For this review, take the finished solid that the model builds, in its own axes (mm). A direction names the side the tool comes from. Coordinates: 2 decimals unless noted, no trailing zeros. Loops run counter-clockwise (first coordinate to the right, second up) from the corner with the lowest first, then second, coordinate; pieces in that order, holes last.
1. Mouldability with a two-part tool opening along Y and no side actions: class faces 3 (the face through (57, 61, 3.2)), 4 (the face through (130.22, 2.99, 1.58)), 5 (the face through (-31.069, 93.114, 1.578)), 6 (the face through (96.05, 4.46, 1.58)) as pulls with the +Y half, pulls with the -Y half, needs draft (parallel to the pull), parting line crosses it, or undercut.
2. Take a section at B-B, the plane y = 3.81. State the section outline as (x, z) points, then the cut area to 3 significant figures.
3. Take a section at C-C, the plane x = 108.5. State the section outline as (y, z) points, then the cut area to 3 significant figures.
4. To check wall thickness, follow probe 1 along Y at (x, z) = (100.5, 2.95); probe 2 along X at (y, z) = (28.5, 1.3); probe 3 along Y at (x, z) = (63, 0.5). State the ranges of each line that lie inside material, in increasing order.
5. Clearance check with a flat-ended pin moving along its axis: P1, Ø1, axis at x = 13.5, z = 1, coming from the +Y side. State where the tip first meets the part, or that it passes through.
6. Machinability: for faces 1 (the face through (-11.48, 3.11, 1.58)), 2 (the face through (72.58, 67.22, 1.62)), which of the approach directions +Z, -Z, +X, -X, +Y, -Y give a long, thin tool a straight path to every point of the face, cutting with its end or side? Answer none if there is none.
7. Take a section at D-D, the plane x = 12.5. State the section outline as (y, z) points, then the cut area to 3 significant figures.
8. Take a section at A-A, the plane x = 81. State the section outline as (y, z) points, then the cut area to 3 significant figures.
```python
from build123d import *

# Parameters (mm, degrees)
SKETCH1_R           = 3.429
SKETCH1_R_2         = 2.54
BOSS_EXTRUDE1_DEPTH = 3.2004
SKETCH2_R           = 2.159
CUT_EXTRUDE1_DEPTH  = 3.2004
CUT_EXTRUDE8_DEPTH  = 3.2004
SKETCH11_W          = 107.95
SKETCH11_H          = 3.2512
CUT_EXTRUDE9_DEPTH  = 3.2004
SKETCH12_R          = 1.1303
CUT_EXTRUDE11_DEPTH = 3.2004
SKETCH13_R          = 2.2479
CUT_EXTRUDE12_DEPTH = 3.2004
BOSS_EXTRUDE2_DEPTH = 3.2004


with BuildPart() as part:
    # Sketch1 → Boss-Extrude1 (new body)
    with BuildSketch(Plane.XY):
        with BuildLine():
            Line((0, 0), (120.015, 0))
            ThreePointArc((120.015, 0), (130.351788397, 3.075697789), (137.325636158, 11.302152593))
            Line((137.325636158, 11.302152593), (155.257499999, 52.11572))
            ThreePointArc((155.257499999, 52.11572), (157.462147967, 67.664529981), (151.26869294, 82.095991421))
            ThreePointArc((151.26869294, 82.095991421), (55.081013593, 128.103082212), (-41.106665754, 82.095991421))
            ThreePointArc((-41.106665754, 82.095991421), (-46.904819593, 67.459968464), (-43.385473773, 52.11572))
            Line((-43.385473773, 52.11572), (-19.648099871, 11.302152593))
            ThreePointArc((-19.648099871, 11.302152593), (-11.333429333, 3.027112684), (0, 0))
        make_face()
        with Locations((120.015, 18.90776)):
            Circle(SKETCH1_R, mode=Mode.SUBTRACT)
        with Locations((0, 18.90776)):
            Circle(SKETCH1_R_2, mode=Mode.SUBTRACT)
        with Locations((19.734727626, 25.566426992)):
            Circle(SKETCH1_R_2, mode=Mode.SUBTRACT)
        with Locations((99.400822531, 30.809360911)):
            Circle(SKETCH1_R_2, mode=Mode.SUBTRACT)
    extrude(amount=BOSS_EXTRUDE1_DEPTH)

    # Sketch2 → Cut-Extrude1 (cut)
    with BuildSketch(Plane(origin=(0, 0, 0), x_dir=(-1, 0, 0), z_dir=(0, 0, -1))):
        with Locations((-92.0115, 52.115719911)):
            Circle(SKETCH2_R)
        with Locations((-28.0035, 52.115719911)):
            Circle(SKETCH2_R)
        with Locations((-98.1075, 3.81)):
            Circle(SKETCH2_R)
        with Locations((-21.9075, 3.81)):
            Circle(SKETCH2_R)
    extrude(amount=-CUT_EXTRUDE1_DEPTH, mode=Mode.SUBTRACT)

    # Sketch10 → Cut-Extrude8 (cut)
    with BuildSketch(Plane(origin=(0, 0, 0), x_dir=(-1, 0, 0), z_dir=(0, 0, -1))):
        with BuildLine():
            Line((-34.3535, 78.785719911), (-21.6535, 78.785719911))
            ThreePointArc((-21.6535, 78.785719911), (-18.4785, 75.610719911), (-21.6535, 72.435719911))
            Line((-21.6535, 72.435719911), (-34.3535, 72.435719911))
            ThreePointArc((-34.3535, 72.435719911), (-37.5285, 75.610719911), (-34.3535, 78.785719911))
        make_face()
    extrude(amount=-CUT_EXTRUDE8_DEPTH, mode=Mode.SUBTRACT)

    # Sketch11 → Cut-Extrude9 (cut)
    with BuildSketch(Plane(origin=(0, 0, 0), x_dir=(-1, 0, 0), z_dir=(0, 0, -1))):
        with Locations((-60.0075, 46.680119911)):
            Rectangle(SKETCH11_W, SKETCH11_H)
    extrude(amount=-CUT_EXTRUDE9_DEPTH, mode=Mode.SUBTRACT)

    # Sketch12 → Cut-Extrude11 (cut)
    with BuildSketch(Plane.XY.offset(3.2004)):
        with Locations((112.438115095, 24.679799513)):
            Circle(SKETCH12_R)
        with Locations((127.591884905, 13.135720487)):
            Circle(SKETCH12_R)
        with BuildLine():
            Line((78.9305, 73.70572), (104.3305, 73.70572))
            ThreePointArc((104.3305, 73.70572), (110.6805, 67.35572), (104.3305, 61.00572))
            Line((104.3305, 61.00572), (78.9305, 61.00572))
            ThreePointArc((78.9305, 61.00572), (72.5805, 67.35572), (78.9305, 73.70572))
        make_face()
        with BuildLine():
            Line((78.9305, 22.08276), (97.9805, 22.08276))
            ThreePointArc((97.9805, 22.08276), (101.1555, 18.90776), (97.9805, 15.73276))
            Line((97.9805, 15.73276), (78.9305, 15.73276))
            ThreePointArc((78.9305, 15.73276), (75.7555, 18.90776), (78.9305, 22.08276))
        make_face()
    extrude(amount=-CUT_EXTRUDE11_DEPTH, mode=Mode.SUBTRACT)

    # Sketch13 → Cut-Extrude12 (cut)
    with BuildSketch(Plane.XY.offset(3.2004)):
        with Locations((-3.91433865, 18.224067698)):
            Circle(SKETCH13_R)
        with Locations((142.479014632, 18.224067698)):
            Circle(SKETCH13_R)
    extrude(amount=-CUT_EXTRUDE12_DEPTH, mode=Mode.SUBTRACT)

    # Sketch15 → Boss-Extrude2 (add)
    with BuildSketch(Plane(origin=(0, 0, 0), x_dir=(-1, 0, 0), z_dir=(0, 0, -1))):
        with BuildLine():
            Line((-83.804619008, 124.717903233), (20.105573884, 102.592791936))
            ThreePointArc((20.105573884, 102.592791936), (13.448555564, 111.243555983), (11.985080527, 122.060665224))
            ThreePointArc((11.985080527, 122.060665224), (-2.230930753, 150.611793243), (-34.052645192, 148.457639579))
            ThreePointArc((-34.052645192, 148.457639579), (-57.674180086, 133.958784174), (-83.804619008, 124.717903233))
        make_face()
    extrude(amount=-BOSS_EXTRUDE2_DEPTH)


solid = part.part
```
Results list:
1. face 3: needs draft
1. face 4: pulls with the -Y half
1. face 5: pulls with the +Y half
1. face 6: undercut
2. outline: (-12.6, 0) - (19.75, 0) - (19.75, 3.2) - (-12.6, 3.2) - close; (24.07, 0) - (95.95, 0) - (95.95, 3.2) - (24.07, 3.2) - close; (100.27, 0) - (131.4, 0) - (131.4, 3.2) - (100.27, 3.2) - close
2. area: 433 mm2
3. outline: (0, 0) - (45.05, 0) - (45.05, 3.2) - (0, 3.2) - close; (48.31, 0) - (62.57, 0) - (62.57, 3.2) - (48.31, 3.2) - close; (72.15, 0) - (115.96, 0) - (115.96, 3.2) - (72.15, 3.2) - close
3. area: 330 mm2
4. probe 1: y = 0 to 16.98, 20.84 to 28.52, 33.1 to 45.05, 48.31 to 61.01, 73.71 to 119.45
4. probe 2: x = -29.65 to 98.34, 100.46 to 144.88
4. probe 3: y = 0 to 45.05, 48.31 to 131.56
5. P1: stops at y = 154.31
6. face 1: +Z, -Z, -X, -Y
6. face 2: +Z, -Z
7. outline: (0, 0) - (45.05, 0) - (45.05, 3.2) - (0, 3.2) - close; (48.31, 0) - (154.14, 0) - (154.14, 3.2) - (48.31, 3.2) - close
7. area: 483 mm2
8. outline: (0, 0) - (15.73, 0) - (15.73, 3.2) - (0, 3.2) - close; (22.08, 0) - (45.05, 0) - (45.05, 3.2) - (22.08, 3.2) - close; (48.31, 0) - (61.01, 0) - (61.01, 3.2) - (48.31, 3.2) - close; (73.71, 0) - (125.42, 0) - (125.42, 3.2) - (73.71, 3.2) - close
8. area: 330 mm2
